from build123d import *

# Parameters (mm, degrees)
CONG_1_R                = 0.1
ENL_V_MAT_EXTRU_1_DEPTH = 0.5


with BuildPart() as part:
    # Esquisse1 → Révolution1 (revolve)
    with BuildSketch(Plane.XY):
        with BuildLine():
            Line((2.2, 0), (1.1, 0))
            Line((1.1, 0), (1.1, -16.5))
            Line((1.1, -16.5), (0, -18))
            Line((0, -18), (0, 1.392961166))
            ThreePointArc((0, 1.392961166), (1.301954378, 1.015441113), (2.2, 0))
        make_face()
    revolve(axis=Axis((0, 3.800054794, 0), (0, -1, 0)))

    # Congé1
    cong_1_edges = [part.edges().sort_by_distance(p)[0] for p in [
        (-2.2, 0, 0),
    ]]
    fillet(cong_1_edges, radius=CONG_1_R)

    # Esquisse2 → Enlèv. mat.-Extru.1 (cut, symmetric)
    with BuildSketch(Plane(origin=(0, 1.15653742, 0), x_dir=(-1, 0, 0), z_dir=(0, 1, 0))):
        Polygon((-0.361948003, 1.140760916), (0.37159995, 1.140760916), (0.37159995, 0.37038863), (1.141972235, 0.37038863), (1.141972235, -0.363159322), (0.37159995, -0.363159322), (0.37159995, -1.133531608), (-0.361948003, -1.133531608), (-0.361948003, -0.363159322), (-1.132320288, -0.363159322), (-1.132320288, 0.37038863), (-0.361948003, 0.37038863), align=None)
    extrude(amount=ENL_V_MAT_EXTRU_1_DEPTH, both=True, mode=Mode.SUBTRACT)


solid = part.part
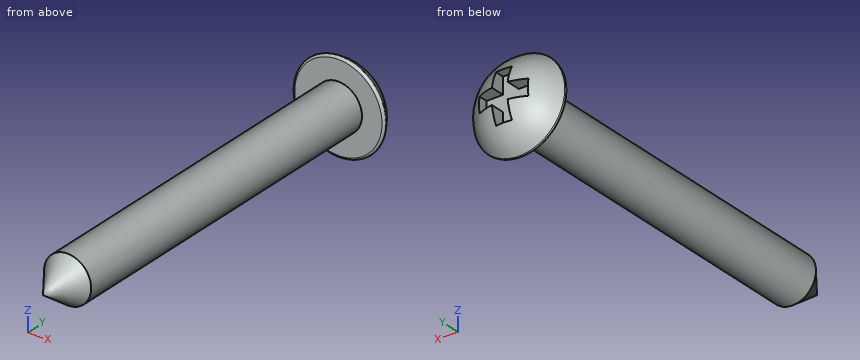
Check sheet for the modelled part. Datum: model origin and axes. Units: mm. Give positions to 0.01 mm unless a question says otherwise; leave off trailing zeros. Loops run counter-clockwise (first coordinate to the right, second up) from the corner with the lowest first, then second, coordinate; pieces in that order, holes last. Notation, with made-up numbers: M 64.25,15 L 80.25,15 A15 ccw 80.25,28 Z; hole C -10.75,61.5 d3. An arc over 180 degrees is marked long. Answer as a JSON object with one key per item and string values. Group by question number.
Q1. Cross-section at A-A on y = -10. Record the cut outline in (x, z).
Q2. Go/stop test with flat-tipped pins: P1, Ø1.5, axis at x = -0.5, z = -1.5, coming from the -Y side; P2, Ø0.5, axis at x = 1, y = 1, coming from the -Z side; P3, Ø0.7, axis at x = 0.5, y = 1, coming from the +Z side. Record where each tip stops, or that it passes through.
Q3. Material ranges on line 1 along Z through (x, y) = (-0.1, -11.25); line 2 along Z through (x, y) = (0.7, -16.75); line 3 along Y through (x, z) = (-1.6, 1.05), recorded low to high. Write a range as [from, to].
Evaluation:
{
 "1": {"outline": "C 0,0 d2.2"},
 "2": {"P1": "stops at y = -16.87", "P2": "stops at z = -1.35", "P3": "stops at z = 1.69"},
 "3": {"line 1": "z = [-1.1, 1.1]", "line 2": "z = [-0.59, 0.59]", "line 3": "y = [0, 0.46]"}
}
